from build123d import *

# Parameters (mm, degrees)
SKETCH_1_R           = 16
EXTRUDE_1_DEPTH      = 80
SKETCH_2_R           = 150
EXTRUDE_2_DEPTH      = 17
SKETCH_3_W           = 8
SKETCH_3_H           = 8
EXTRUDE_3_DEPTH      = 0.1
EXTRUDE_3_DEPTH_BACK = 45
SKETCH_4_R           = 115
SKETCH_4_R_2         = 109
EXTRUDE_4_DEPTH      = 4
SKETCH_5_R           = 109
SKETCH_5_R_2         = 30
CUT_EXTRUDE_1_DEPTH  = 8
CHAMFER_1_SIZE       = 1
SKETCH_6_R           = 7.5
CUT_EXTRUDE_2_DEPTH  = 18
SKETCH_7_R           = 95
EXTRUDE_5_DEPTH      = 39
SKETCH_8_R           = 98
EXTRUDE_6_DEPTH      = 199
SKETCH_9_R           = 101
EXTRUDE_7_DEPTH      = 100
CHAMFER_2_SIZE       = 42
EXTRUDE_8_DEPTH      = 170
CUT_EXTRUDE_3_REACH  = 264
SKETCH_11_R          = 6
SKETCH_12_W          = 80
SKETCH_12_H          = 85
EXTRUDE_9_DEPTH      = 173
SKETCH_13_R          = 20
EXTRUDE_10_DEPTH     = 103
CHAMFER_3_SIZE       = 1
SKETCH_15_R          = 6
SKETCH_16_R          = 10
EXTRUDE_11_DEPTH     = 14
EXTRUDE_12_DEPTH     = 14
SKETCH_18_R          = 6
CUT_EXTRUDE_4_DEPTH  = 14


with BuildPart() as part:
    # Эскиз1 → Вытянуть1 (new body)
    with BuildSketch(Plane.XY):
        Circle(SKETCH_1_R)
    extrude(amount=EXTRUDE_1_DEPTH)

    # Эскиз2 → Вытянуть2 (add)
    with BuildSketch(Plane(origin=(0, 0, 0), x_dir=(-1, 0, 0), z_dir=(0, 0, -1))):
        Circle(SKETCH_2_R)
    extrude(amount=EXTRUDE_2_DEPTH)

    # Эскиз3 → Вытянуть3 (add, two sides)
    with BuildSketch(Plane.XY.offset(80)) as extrude_3_sk:
        with Locations((0, 15)):
            Rectangle(SKETCH_3_W, SKETCH_3_H)
    extrude(amount=EXTRUDE_3_DEPTH)
    extrude(extrude_3_sk.sketch, amount=-EXTRUDE_3_DEPTH_BACK)

    # Эскиз4 → Вытянуть4 (add)
    with BuildSketch(Plane.XY):
        with Locations(Location((0, 0, 0), (0, 0, 180))):  # turned: the seam where the file's is
            Circle(SKETCH_4_R)
        Circle(SKETCH_4_R_2, mode=Mode.SUBTRACT)
    extrude(amount=EXTRUDE_4_DEPTH)

    # Эскиз5 → Вырез-Вытянуть1 (cut)
    with BuildSketch(Plane.XY):
        Circle(SKETCH_5_R)
        Circle(SKETCH_5_R_2, mode=Mode.SUBTRACT)
    extrude(amount=-CUT_EXTRUDE_1_DEPTH, mode=Mode.SUBTRACT)

    # Фаска1
    chamfer_1_edges = [part.edges().sort_by_distance(p)[0] for p in [
        (115, 0, 4),
        (-30, 0, 0),
        (-9.797958971, -12.649110641, 80),
    ]]
    chamfer(chamfer_1_edges, length=CHAMFER_1_SIZE)

    # Эскиз6 → Вырез-Вытянуть2 (cut, through all)
    with BuildSketch(Plane.XY):
        with Locations((-50.705554788, 122.414038058)):
            Circle(SKETCH_6_R)
        with Locations((50.705554788, 122.414038058)):
            Circle(SKETCH_6_R)
        with Locations((122.414038058, 50.705554788)):
            Circle(SKETCH_6_R)
        with Locations((122.414038058, -50.705554788)):
            Circle(SKETCH_6_R)
        with Locations((50.705554788, -122.414038058)):
            Circle(SKETCH_6_R)
        with Locations((-50.705554788, -122.414038058)):
            Circle(SKETCH_6_R)
        with Locations((-122.414038058, -50.705554788)):
            Circle(SKETCH_6_R)
        with Locations((-122.414038058, 50.705554788)):
            Circle(SKETCH_6_R)
    extrude(amount=-CUT_EXTRUDE_2_DEPTH, mode=Mode.SUBTRACT)

    # Эскиз7 → Вытянуть5 (add)
    with BuildSketch(Plane(origin=(0, 0, -17), x_dir=(-1, 0, 0), z_dir=(0, 0, -1))):
        Circle(SKETCH_7_R)
    extrude(amount=EXTRUDE_5_DEPTH)

    # Эскиз8 → Вытянуть6 (add)
    with BuildSketch(Plane(origin=(0, 0, -56), x_dir=(-1, 0, 0), z_dir=(0, 0, -1))):
        Circle(SKETCH_8_R)
    extrude(amount=EXTRUDE_6_DEPTH)

    # Эскиз9 → Вытянуть7 (add)
    with BuildSketch(Plane(origin=(0, 0, -255), x_dir=(-1, 0, 0), z_dir=(0, 0, -1))):
        Circle(SKETCH_9_R)
    extrude(amount=EXTRUDE_7_DEPTH)

    # Фаска2
    chamfer_2_edges = [part.edges().sort_by_distance(p)[0] for p in [
        (101, 0, -355),
    ]]
    chamfer(chamfer_2_edges, length=CHAMFER_2_SIZE)

    # Эскиз10 → Вытянуть8 (add)
    with BuildSketch(Plane.XY.offset(-56)):
        Polygon((-110, -112), (-71.917096231, -112), (-51.440399562, -76.533320997), (-63.564755215, -69.533320997), (-80, -98), (-110, -98), align=None)
        Polygon((110, -98), (110, -112), (71.917096231, -112), (51.440399562, -76.533320997), (63.564755215, -69.533320997), (80, -98), align=None)
    extrude(amount=-EXTRUDE_8_DEPTH)

    # Эскиз11 → Вырез-Вытянуть3 (cut, up to next)
    with BuildSketch(Plane.XZ.offset(112), mode=Mode.PRIVATE) as cut_extrude_3_sk1:
        with Locations(Location((95, -70, 0), (0, 0, 270))):  # turned: the seam where the file's is
            Circle(SKETCH_11_R)
    cut_extrude_3_tool1 = extrude(cut_extrude_3_sk1.sketch, amount=-CUT_EXTRUDE_3_REACH, mode=Mode.PRIVATE) & part.part
    add(cut_extrude_3_tool1.solids().sort_by_distance((95, -112, -70))[0], mode=Mode.SUBTRACT)
    # Эскиз11 → Вырез-Вытянуть3 (cut, up to next)
    with BuildSketch(Plane.XZ.offset(112), mode=Mode.PRIVATE) as cut_extrude_3_sk2:
        with Locations(Location((-95, -70, 0), (0, 0, 270))):  # turned: the seam where the file's is
            Circle(SKETCH_11_R)
    cut_extrude_3_tool2 = extrude(cut_extrude_3_sk2.sketch, amount=-CUT_EXTRUDE_3_REACH, mode=Mode.PRIVATE) & part.part
    add(cut_extrude_3_tool2.solids().sort_by_distance((-95, -112, -70))[0], mode=Mode.SUBTRACT)
    # Эскиз11 → Вырез-Вытянуть3 (cut, up to next)
    with BuildSketch(Plane.XZ.offset(112), mode=Mode.PRIVATE) as cut_extrude_3_sk3:
        with Locations(Location((95, -210, 0), (0, 0, 270))):  # turned: the seam where the file's is
            Circle(SKETCH_11_R)
    cut_extrude_3_tool3 = extrude(cut_extrude_3_sk3.sketch, amount=-CUT_EXTRUDE_3_REACH, mode=Mode.PRIVATE) & part.part
    add(cut_extrude_3_tool3.solids().sort_by_distance((95, -112, -210))[0], mode=Mode.SUBTRACT)
    # Эскиз11 → Вырез-Вытянуть3 (cut, up to next)
    with BuildSketch(Plane.XZ.offset(112), mode=Mode.PRIVATE) as cut_extrude_3_sk4:
        with Locations(Location((-95, -210, 0), (0, 0, 270))):  # turned: the seam where the file's is
            Circle(SKETCH_11_R)
    cut_extrude_3_tool4 = extrude(cut_extrude_3_sk4.sketch, amount=-CUT_EXTRUDE_3_REACH, mode=Mode.PRIVATE) & part.part
    add(cut_extrude_3_tool4.solids().sort_by_distance((-95, -112, -210))[0], mode=Mode.SUBTRACT)

    # Эскиз12 → Вытянуть9 (add)
    with BuildSketch(Plane(origin=(0, 0, 0), x_dir=(1, 0, 0), z_dir=(0, 1, 0))):
        with Locations((0, 99.5)):
            Rectangle(SKETCH_12_W, SKETCH_12_H)
    extrude(amount=EXTRUDE_9_DEPTH)

    # Эскиз13 → Вытянуть10 (add)
    with BuildSketch(Plane(origin=(0, 0, 0), x_dir=(1, 0, 0), z_dir=(0, 1, 0))):
        with Locations(Location((0, 170, 0), (0, 0, 90))):  # turned: the seam where the file's is
            Circle(SKETCH_13_R)
    extrude(amount=EXTRUDE_10_DEPTH)

    # Фаска3
    chamfer_3_edges = [part.edges().sort_by_distance(p)[0] for p in [
        (0, 103, -150),
    ]]
    chamfer(chamfer_3_edges, length=CHAMFER_3_SIZE)

    # По траектории1: sweep along a path in Эскиз14
    with BuildLine(Plane.XY.offset(-170)) as sweep_1_path:
        CenterArc((0, 128), 25, 0, 360)
    # Эскиз15 → По траектории1 (sweep)
    with BuildSketch(Plane(origin=(0, 0, 0), x_dir=(0, 0, -1), z_dir=(1, 0, 0))):
        with Locations((170, 153)):
            Circle(SKETCH_15_R)
    sweep(path=sweep_1_path.line)

    # Эскиз16 → Вытянуть11 (add)
    with BuildSketch(Plane(origin=(40, 0, 0), x_dir=(0, 0, -1), z_dir=(1, 0, 0))):
        with Locations(Location((99.5, 138, 0), (0, 0, 180))):  # turned: the seam where the file's is
            Circle(SKETCH_16_R)
    extrude(amount=EXTRUDE_11_DEPTH)

    # Эскиз17 → Вытянуть12 (add)
    with BuildSketch(Plane(origin=(54, 0, 0), x_dir=(0, 0, -1), z_dir=(1, 0, 0))):
        Polygon((99.5, 159.36195996), (81, 148.68097998), (81, 127.31902002), (99.5, 116.63804004), (118, 127.31902002), (118, 148.68097998), align=None)
    extrude(amount=EXTRUDE_12_DEPTH)

    # Эскиз18 → Вырез-Вытянуть4 (cut)
    with BuildSketch(Plane(origin=(68, 0, 0), x_dir=(0, 0, -1), z_dir=(1, 0, 0))):
        with Locations((99.5, 138)):
            Circle(SKETCH_18_R)
    extrude(amount=-CUT_EXTRUDE_4_DEPTH, mode=Mode.SUBTRACT)


solid = part.part
Design review of the part built by this model. Coordinates are the model's own, in mm. A direction names the side the tool comes from. Give positions to 0.01 mm unless a question says otherwise; leave off trailing zeros. Order: outer loops, then holes, each group sorted by start corner. A loop starts at its lowest first (then second) coordinate and runs counter-clockwise, first axis right, second up.
1. Add section C-C, the plane z = -277. State the section outline as (x, y) points.
Solution:
outline: circle Ø202 at (0, 0)
2. Add section B-B, the plane z = -170. State the section outline as (x, y) points, then the cut area to 3 significant figures.
Solution:
outline: (-110, -112) - (-71.92, -112) - (-54.34, -81.55) arc R98 ccw to (54.34, -81.55) - (71.92, -112) - (110, -112) - (110, -98) - (80, -98) - (65.5, -72.89) arc R98 ccw to (20, 95.94) - (20, 102) - (19, 103) - (18.33, 103) arc R31 ccw (long way) to (-18.33, 103) - (-19, 103) - (-20, 102) - (-20, 95.94) arc R98 ccw to (-65.5, -72.89) - (-80, -98) - (-110, -98) - close; hole circle Ø38 at (0, 128)
area: 34,000 mm2
3. Add section A-A, the plane z = -70. State the section outline as (x, y) points, then the cut area to 3 significant figures.
Solution:
outline: (-110, -112) - (-101, -112) - (-101, -98) - (-110, -98) - close; (-89, -112) - (-71.92, -112) - (-54.34, -81.55) arc R98 ccw to (54.34, -81.55) - (71.92, -112) - (89, -112) - (89, -98) - (80, -98) - (65.5, -72.89) arc R98 ccw to (40, 89.47) - (40, 173) - (-40, 173) - (-40, 89.47) arc R98 ccw to (-65.5, -72.89) - (-80, -98) - (-89, -98) - close; (101, -112) - (110, -112) - (110, -98) - (101, -98) - close
area: 37,900 mm2
4. Tool access review of faces 5 (the flat face through (54, 138, -99)), 6 (the flat face through (56, 101, 0)), 7 (the flat face through (23.9, -92.1, -56)), 8 (the cylindrical face through (-124.04, -58.027, -8.381)), 9 (the flat face through (-110, -105, -140)): name each direction out of +Z, -Z, +X, -X, +Y, -Y from which nothing blocks a thin tool from reaching the whole face with its end or side.
Solution:
face 5: +X
face 6: +Z
face 7: none
face 8: +Z, -Z
face 9: -Z, -X, +Y, -Y
5. For pin 1 Ø1 at (y, z) = (83.5, -124) entering from -X; pin 2 Ø19 at (x, z) = (95, -210) entering from +Y; pin 3 Ø15.5 at (x, z) = (95, -70) entering from -Y, all flat-tipped, find the tip position at first contact; note any pin that passes through.
Solution:
pin 1: stops at x = -52.11
pin 2: stops at y = 47.89
pin 3: stops at y = -112
6. Mouldability with a two-part tool opening along Y and no side actions: class faces 1 (the flat face through (60.902, 154.096, -90.38)), 2 (the cylindrical face through (49.08, 115.092, -8.381)), 3 (the flat face through (-63.25, -96.99, -139.81)), 4 (the flat face through (-40, 131, -99)) as +Y half, -Y half, draft (parallel to the pull), parting line (faces both ways), or undercut.
Solution:
face 1: +Y half
face 2: undercut
face 3: -Y half
face 4: draft
7. To check wall thickness, follow L1, parallel to Z at x = -12, y = 26.5; L2, parallel to Y at x = -3.5, z = -53; L3, parallel to X at y = -102, z = -210. State the ranges of each line that lie inside material, in increasing order.
Solution:
L1: z = -355 to -0.09
L2: y = -94.94 to 94.94
L3: x = -110 to -101, -89 to -66.14, 66.14 to 89, 101 to 110
